Source: CAD feature listing. Evaluate the final solid. Frame: model axes, mm. A direction names the side the tool comes from. Round coordinates to 2 decimals unless told otherwise and drop trailing zeros. Order: outer loops, then holes, each group sorted by start corner. A loop starts at its lowest first (then second) coordinate and runs counter-clockwise, first axis right, second up. Notation, with made-up numbers: M 49,20.5 L 92,20.5 A14 ccw 92,29.5 Z; hole C 85.5,-8.75 d10. An arc over 180 degrees is marked long. Answer as CSV lines item,"result". Start each with the question number.
Item 1: Pull-direction query (X, two-part tool) for faces 3 (the face through (128.91, -72.49, -12.52)), 4 (the face through (296.28, -31.44, -12.52)), 5 (the face through (143.181, 47.343, -12.522)), 6 (the face through (120.6, 99.5, -12.5)); classes: +X half, -X half, draft (parallel to the pull), parting line (faces both ways), or undercut.
Item 2: Section query C-C on y = 60. Return the cut outline in (x, z), plus the area to 3 significant figures.
Item 3: Section query A-A on z = -11.5. Return the cut outline in (x, y).
Item 4: Section query D-D on x = 20. Return the cut outline in (y, z), plus the area to 3 significant figures.
Item 5: Line query: line 1 (X direction, y = 17, z = -10.5); line 2 (X direction, y = 26, z = -10.25); line 3 (Y direction, x = 152, z = -12.5). Output: solid intervals per line, ascending. Write a range as [from, to].
Item 6: First-contact query: P1, Ø2, axis at x = 60, z = -15.5, coming from the +Y side; P2, Ø23, axis at x = 241.5, y = -172.81, coming from the +Z side; P3, Ø1.5, axis at x = 161, z = -18, coming from the -Y side; P4, Ø2, axis at x = 137.5, z = -18.5, coming from the -Y side. Flat tips, straight axial feed; report the tip coordinate or a pass-through.
Item 7: Set-up query: faces 1 (the face through (243.798, 85.357, -12.522)), 2 (the face through (-42.787, 4.498, -12.522)). Return all of +Z, -Z, +X, -X, +Y, -Y with unobstructed straight access to the full face (end or side cutting, diameter ignored); none if empty.
Item 8: Section query B-B on x = 130. Return the cut outline in (y, z).
from build123d import *

# Parameters (mm, degrees)
SKETCH1_R      = 12.7
EXTRUDE1_DEPTH = 25.4


with BuildPart() as part:
    # Sketch1 → Extrude1 (new body)
    with BuildSketch(Plane.XY):
        Polygon((-44.980643346, -17.930846203), (239.040212224, -221.173843873), (279.515997466, -202.802308581), (313.519168805, 144.788466381), (277.371059915, 170.655756994), (-40.652966993, 26.307979701), align=None)
        Circle(SKETCH1_R, mode=Mode.SUBTRACT)
        with Locations((270.409306565, 122.735954077)):
            Circle(SKETCH1_R, mode=Mode.SUBTRACT)
        with Locations((241.497107471, -172.813351867)):
            Circle(SKETCH1_R, mode=Mode.SUBTRACT)
        Polygon((44.892749422, -12.367036283), (215.305262763, -134.312834884), (229.76090035, -127.75157228), (250.162803153, 80.802892697), (237.252764264, 90.041210773), (46.438348119, 3.432544398), align=None, mode=Mode.SUBTRACT)
    extrude(amount=-EXTRUDE1_DEPTH)


solid = part.part
Results:
1,face 3,"undercut"
1,face 4,"+X half"
1,face 5,"undercut"
1,face 6,"-X half"
2,outline,"M 33.58,-25.4 L 171.07,-25.4 L 171.07,0 L 33.58,0 Z; M 248.13,-25.4 L 305.22,-25.4 L 305.22,0 L 248.13,0 Z"
2,area,"4,940 mm^2"
3,outline,"M -44.98,-17.93 L 239.04,-221.17 L 279.52,-202.8 L 313.52,144.79 L 277.37,170.66 L -40.65,26.31 Z; hole C 0,0 d25.4; hole M 44.89,-12.37 L 215.31,-134.31 L 229.76,-127.75 L 250.16,80.8 L 237.25,90.04 L 46.44,3.43 Z; hole C 241.5,-172.81 d25.4; hole C 270.41,122.74 d25.4"
4,outline,"M -64.43,-25.4 L 53.84,-25.4 L 53.84,0 L -64.43,0 Z"
4,area,"3,000 mm^2"
5,line 1,"[-41.56, 76.33], [243.92, 301.02]"
5,line 2,"[-40.68, 96.16], [244.8, 301.9]"
5,line 3,"[-158.89, -89.01], [51.35, 113.75]"
6,P1,"y = 72.45"
6,P2,"through"
6,P3,"y = -165.87"
6,P4,"y = -149.23"
7,face 1,"+Z, -Z"
7,face 2,"+Z, -Z, -X, +Y"
8,outline,"M -143.15,-25.4 L -73.27,-25.4 L -73.27,0 L -143.15,0 Z; M 41.36,-25.4 L 103.77,-25.4 L 103.77,0 L 41.36,0 Z"
